Model file for the job. Use its own axes, mm. A direction names the side the tool comes from. Round coordinates to 2 decimals unless told otherwise and drop trailing zeros. Loops run counter-clockwise (first coordinate to the right, second up) from the corner with the lowest first, then second, coordinate; pieces in that order, holes last. Notation, with made-up numbers: (72, 39) - (118, 39) arc R6 cw to (118, 48) - close; hole circle Ø5 at (51, 14.5). An arc over 180 degrees is marked (long way). Use one line per item in the form item = value.
from build123d import *

# Parameters (mm, degrees)
F1_DEPTH       = 60
F2_R           = 0.8
F4_DEPTH       = 12.5
F6_D           = 3.5
F6_CSINK_D     = 6.5
F6_CSINK_ANGLE = 90


with BuildPart() as f1:
    # F0 (on Front) → F1 (new body, symmetric)
    with BuildSketch(Plane.XZ):
        Polygon((37.55, 0), (0, 0), (-37.55, 0), (-37.55, 10), (-34.55, 13), (-40.05, 13), (-40.05, -2), (0, -2), (40.05, -2), (40.05, 13), (34.55, 13), (37.55, 10), align=None)
    extrude(amount=F1_DEPTH, both=True)

    # F2
    f2_edges = [f1.edges().sort_by_distance(p)[0] for p in [
        (-34.55, 0, 13),
        (34.55, 0, 13),
    ]]
    fillet(f2_edges, radius=F2_R)

    # F3 (on face) → F4 (intersect, symmetric)
    with BuildSketch(Plane.XY):
        Polygon((-20.05, -8), (40.05, -60), (40.05, -48), (20.05, -30.695507), (20.05, 0), (20.05, 30.695507), (40.05, 48), (40.05, 60), (-20.05, 8), (-40.05, 8), (-40.05, 0), (-40.05, -8), align=None)
    extrude(amount=F4_DEPTH, both=True, mode=Mode.INTERSECT)

    # F6 (through all)
    with Locations(Plane.XY):
        with Locations((-5, 0)):
            CounterSinkHole(F6_D / 2, F6_CSINK_D / 2, counter_sink_angle=F6_CSINK_ANGLE)


solid = f1.part
1. Wall check: probe 1 along X at (y, z) = (0, -1.7); probe 2 along Z at (x, y) = (-10, 7.5); probe 3 along Y at (x, z) = (-5, -1.65). Give the ranges that are in metal, low to high.
Geometry check:
probe_1 = -40.05 to -6.75, -3.25 to 20.05
probe_2 = -2 to 0
probe_3 = -21.02 to -1.75, 1.75 to 21.02
2. Flat gauge pins, fed straight in: pin 1 (1.6 mm diameter, centred on y = 13, z = -1, fed in from +X); pin 2 (1.5 mm diameter, centred on x = 27, z = 2.5, fed in from +Y); pin 3 (12 mm diameter, centred on x = 9.5, y = 11, fed in from +Z); pin 4 (3 mm diameter, centred on y = 51.5, z = 4.5, fed in from -X). Where does each tip first touch, or does it go through?
Geometry check:
pin_1 = 20.05
pin_2 = through
pin_3 = 0
pin_4 = 37.55
3. Cut at A-A, the plane y = 0. Give the cut face in (x, z), plus the area to 3 significant figures.
Geometry check:
outline = (-40.05, -2) - (-6.75, -2) - (-6.75, -1.5) - (-8.25, 0) - (-37.55, 0) - (-37.55, 10) - (-35.92, 11.63) arc R0.8 ccw to (-35.74, 12.5) - (-40.05, 12.5) - close; (-3.25, -2) - (20.05, -2) - (20.05, 0) - (-1.75, 0) - (-3.25, -1.5) - close
area = 145 mm^2
4. Cut at B-B, the plane x = 26.5. Give the cut face in (y, z), plus the area to 3 significant figures.
Geometry check:
outline = (-48.28, -2) - (-36.28, -2) - (-36.28, 0) - (-48.28, 0) - close; (36.28, -2) - (48.28, -2) - (48.28, 0) - (36.28, 0) - close
area = 48.0 mm^2
5. Cut at C-C, the plane z = 2.25. Give the cut face in (x, y).
Geometry check:
outline = (-40.05, -8) - (-37.55, -8) - (-37.55, 8) - (-40.05, 8) - close; (37.55, -57.84) - (40.05, -60) - (40.05, -48) - (37.55, -45.84) - close; (37.55, 45.84) - (40.05, 48) - (40.05, 60) - (37.55, 57.84) - close
6. Cut at D-D, the plane y = -49.5. Give the cut face in (x, z), plus the area to 3 significant figures.
Geometry check:
outline = (27.91, -2) - (40.05, -2) - (40.05, 12.5) - (35.74, 12.5) arc R0.8 ccw to (35.92, 11.63) - (37.55, 10) - (37.55, 0) - (27.91, 0) - close
area = 58.4 mm^2
7. Tool access for faces 1 (the flat face through (-37.55, 0, 5)), 2 (the flat face through (33.707, 42.512, -0.624)), 3 (the flat face through (-38, 0, 12.5)), 4 (the flat face through (37.55, 52, 5)), 5 (the flat face through (-34, 8, -1)): list every direction of +Z, -Z, +X, -X, +Y, -Y with a clear straight run to the whole face (end or side of a thin tool).
Geometry check:
face_1 = +X, +Y, -Y
face_2 = +Z, -Z, +X
face_3 = +Z, +X, -X, +Y, -Y
face_4 = -X, +Y, -Y
face_5 = +Z, -Z, -X, +Y
8. Pull direction Z, two halves, no side cores. Call faces 6 (the flat face through (38, -52, 12.5)), 7 (the flat face through (37.55, -52, 5)), 8 (the flat face through (-33, -8, -1)): +Z half, -Z half, draft (parallel to the pull), parting line (faces both ways), or undercut.
Geometry check:
face_6 = +Z half
face_7 = undercut
face_8 = draft
